Build history of the part. All positions in model axes, mm. A direction names the side the tool comes from. Round coordinates to 2 decimals unless told otherwise and drop trailing zeros. Loops run counter-clockwise (first coordinate to the right, second up) from the corner with the lowest first, then second, coordinate; pieces in that order, holes last.
from build123d import *

# Parameters (mm, degrees)
SKETCH1_R           = 7.5
BOSS_EXTRUDE1_DEPTH = 49
FILLET1_R           = 10
SKETCH2_R           = 7.25
BOSS_EXTRUDE2_DEPTH = 25
CUT_EXTRUDE1_START  = -15
CUT_EXTRUDE1_DEPTH  = 15


with BuildPart() as part:
    # Sketch1 → Boss-Extrude1 (new body)
    with BuildSketch(Plane.XY):
        with BuildLine():
            ThreePointArc((-7.448470559, -0.877659574), (-7.5, 0), (-7.448470559, 0.877659574))
            Line((-7.448470559, 0.877659574), (-6.755839639, 6.755839639))
            Line((-6.755839639, 6.755839639), (-47.234042553, 1.986258816))
            ThreePointArc((-47.234042553, 1.986258816), (-49, 0), (-47.234042553, -1.986258816))
            Line((-47.234042553, -1.986258816), (-6.755839639, -6.755839639))
            Line((-6.755839639, -6.755839639), (-7.448470559, -0.877659574))
        make_face()
        with BuildLine():
            Line((-1.986258816, 47.234042553), (-6.755839639, 6.755839639))
            Line((-6.755839639, 6.755839639), (-0.877659574, 7.448470559))
            ThreePointArc((-0.877659574, 7.448470559), (0, 7.5), (0.877659574, 7.448470559))
            Line((0.877659574, 7.448470559), (6.755839639, 6.755839639))
            Line((6.755839639, 6.755839639), (1.986258816, 47.234042553))
            ThreePointArc((1.986258816, 47.234042553), (0, 49), (-1.986258816, 47.234042553))
        make_face()
        with BuildLine():
            Line((47.234042553, 1.986258816), (6.755839639, 6.755839639))
            Line((6.755839639, 6.755839639), (7.448470559, 0.877659574))
            ThreePointArc((7.448470559, 0.877659574), (7.487106557, 0.43958549), (7.5, 0))
            ThreePointArc((7.5, 0), (7.487106557, -0.43958549), (7.448470559, -0.877659574))
            Line((7.448470559, -0.877659574), (6.755839639, -6.755839639))
            Line((6.755839639, -6.755839639), (47.234042553, -1.986258816))
            ThreePointArc((47.234042553, -1.986258816), (49, 0), (47.234042553, 1.986258816))
        make_face()
        with BuildLine():
            Line((-0.877659574, -7.448470559), (-6.755839639, -6.755839639))
            Line((-6.755839639, -6.755839639), (-1.986258816, -47.234042553))
            ThreePointArc((-1.986258816, -47.234042553), (0, -49), (1.986258816, -47.234042553))
            Line((1.986258816, -47.234042553), (6.755839639, -6.755839639))
            Line((6.755839639, -6.755839639), (0.877659574, -7.448470559))
            ThreePointArc((0.877659574, -7.448470559), (0, -7.5), (-0.877659574, -7.448470559))
        make_face()
        with BuildLine():
            Line((-6.755839639, 6.755839639), (-7.448470559, 0.877659574))
            ThreePointArc((-7.448470559, 0.877659574), (-5.303300859, 5.303300859), (-0.877659574, 7.448470559))
            Line((-0.877659574, 7.448470559), (-6.755839639, 6.755839639))
        make_face()
        Circle(SKETCH1_R)
        with BuildLine():
            Line((6.755839639, 6.755839639), (0.877659574, 7.448470559))
            ThreePointArc((0.877659574, 7.448470559), (5.303300859, 5.303300859), (7.448470559, 0.877659574))
            Line((7.448470559, 0.877659574), (6.755839639, 6.755839639))
        make_face()
        with BuildLine():
            ThreePointArc((7.448470559, -0.877659574), (5.303300859, -5.303300859), (0.877659574, -7.448470559))
            Line((0.877659574, -7.448470559), (6.755839639, -6.755839639))
            Line((6.755839639, -6.755839639), (7.448470559, -0.877659574))
        make_face()
        with BuildLine():
            ThreePointArc((-0.877659574, -7.448470559), (-5.303300859, -5.303300859), (-7.448470559, -0.877659574))
            Line((-7.448470559, -0.877659574), (-6.755839639, -6.755839639))
            Line((-6.755839639, -6.755839639), (-0.877659574, -7.448470559))
        make_face()
    extrude(amount=BOSS_EXTRUDE1_DEPTH)

    # Fillet1
    fillet1_edges = [part.edges().sort_by_distance(p)[0] for p in [
        (6.755839639, 6.755839639, 24.5),
        (6.755839639, -6.755839639, 24.5),
        (-6.755839639, -6.755839639, 24.5),
        (-6.755839639, 6.755839639, 24.5),
    ]]
    fillet(fillet1_edges, radius=FILLET1_R)

    # Sketch2 → Boss-Extrude2 (add)
    with BuildSketch(Plane(origin=(0, 0, 0), x_dir=(-1, 0, 0), z_dir=(0, 0, -1))):
        with Locations(Location((0, 0, 0), (0, 0, 180))):
            Circle(SKETCH2_R)
    extrude(amount=BOSS_EXTRUDE2_DEPTH)

    # Sketch3 → Cut-Extrude1 (cut)
    with BuildSketch(Plane(origin=(0, 0, -25), x_dir=(-1, 0, 0), z_dir=(0, 0, -1)).offset(CUT_EXTRUDE1_START)):
        with BuildLine():
            Line((6.968679932, -2), (-6.968679932, -2))
            ThreePointArc((-6.968679932, -2), (0, -7.25), (6.968679932, -2))
        make_face()
    extrude(amount=CUT_EXTRUDE1_DEPTH, mode=Mode.SUBTRACT)


solid = part.part
(1) Slice it at D-D on z = -12. List the corners of the cut face in (x, y).
Responses:
outline: (-6.97, -2) - (6.97, -2) arc R7.25 ccw (long way) to start
(2) Which spindle directions (+Z, -Z, +X, -X, +Y, -Y) get a long thin tool onto all of the face, cutting with end or side? Do faces 1 (the face through (-1.57, 7.08, -9.55)), 2 (the face through (0, -2, -17)), 3 (the face through (-8.759, -8.627, 24.843)). Say none if no direction does.
Responses:
face 1: -Z
face 2: -Z, +X, -X, -Y
face 3: +Z, -Z, -X, -Y
(3) Slice it at A-A on z = 2.5. List the corners of the cut face in (x, y), plus the area to 3 significant figures.
Responses:
outline: (-47.23, -1.99) - (-14.59, -5.83) arc R10 cw to (-5.83, -14.59) - (-1.99, -47.23) arc R2 ccw to (1.99, -47.23) - (5.83, -14.59) arc R10 cw to (14.59, -5.83) - (47.23, -1.99) arc R2 ccw to (47.23, 1.99) - (14.59, 5.83) arc R10 cw to (5.83, 14.59) - (1.99, 47.23) arc R2 ccw to (-1.99, 47.23) - (-5.83, 14.59) arc R10 cw to (-14.59, 5.83) - (-47.23, 1.99) arc R2 ccw to start
area: 1,670 mm2
(4) Pin check, flat tips, straight feed: P1, Ø6, axis at y = 38.5, z = 11.5, coming from the -X side; P2, Ø1, axis at x = -10.5, z = 13, coming from the -Y side; P3, Ø8, axis at y = -2.5, z = -17, coming from the +X side. Stop position of each tip, or through.
Responses:
P1: stops at x = -3.37
P2: stops at y = -7.59
P3: stops at x = 7.25
(5) Slice it at B-B on x = 0. List the corners of the cut face in (y, z).
Responses:
outline: (-49, 0) - (-7.25, 0) - (-7.25, -10) - (-2, -10) - (-2, -25) - (7.25, -25) - (7.25, 0) - (49, 0) - (49, 49) - (-49, 49) - close
(6) Slice it at C-C on y = 0. List the corners of the cut face in (x, z), plus the area to 3 significant figures.
Responses:
outline: (-49, 0) - (-7.25, 0) - (-7.25, -25) - (7.25, -25) - (7.25, 0) - (49, 0) - (49, 49) - (-49, 49) - close
area: 5,160 mm2
(7) Probe line 1 (X direction, y = 2, z = -8); line 2 (Z direction, x = -28, y = -1); line 3 (X direction, y = 14.5, z = 4). List the from-to ranges inside material, lowest first.
Responses:
line 1: x = -6.97 to 6.97
line 2: z = 0 to 49
line 3: x = -5.84 to 5.84
